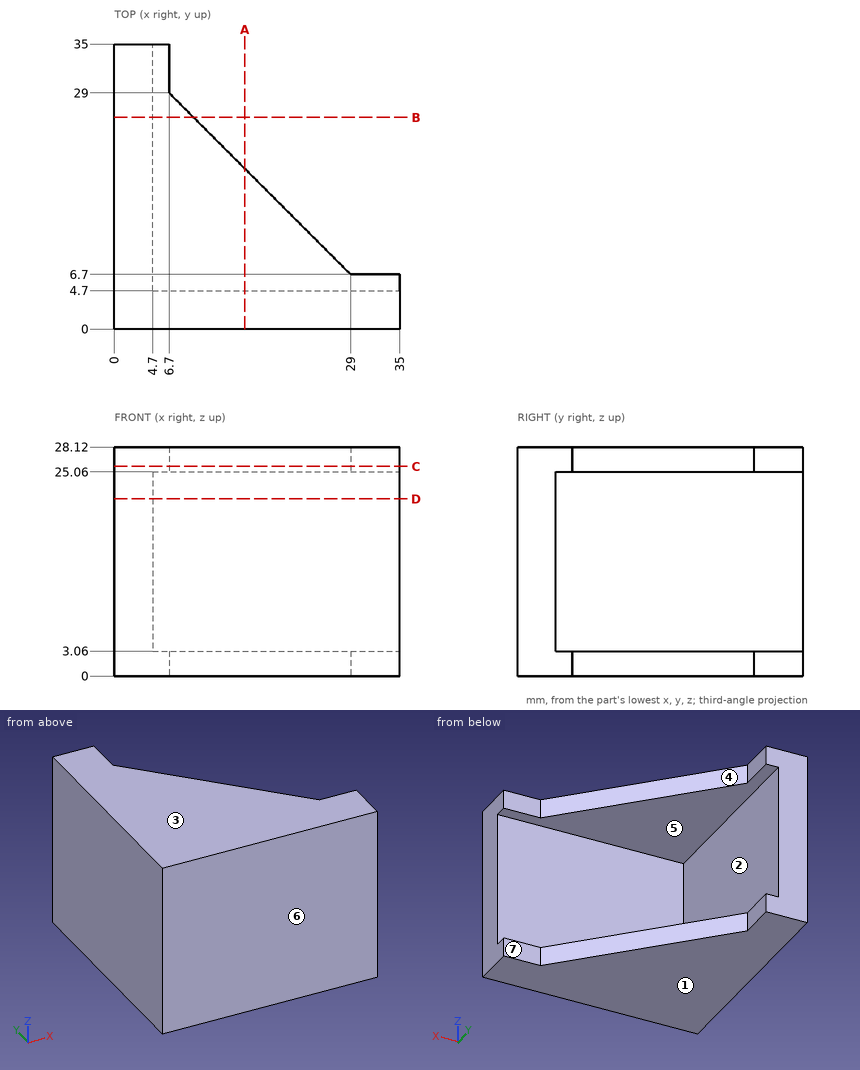
Could you check a few things on this drawing? It's one solid part, dimensions in mm from its lowest x, y, z. A direction names the side the tool comes from. Round coordinates to 2 decimals unless told otherwise and drop trailing zeros. Order: outer loops, then holes, each group sorted by start corner. A loop starts at its lowest first (then second) coordinate and runs counter-clockwise, first axis right, second up. Notation, with made-up numbers: M -25,19.25 L -14,19.25 A12 cw -14,23.25 Z; hole C 78,0.5 d8. An arc over 180 degrees is marked long. Return JSON: item names as keys, results as strings. Group by question number.
1. If we mould it in two halves opening along Z, with no side actions, what happens to the marked faces 1, 2, 3 and 4? For each: pulls with the +Z half, pulls with the -Z half, needs draft (parallel to the pull), parting line crosses it, or undercut.
2. If we section it at A-A on x = 16: List the corners of the cut face in (y, z) for me.
3. If we section it at B-B on y = 26: List the corners of the cut face in (x, z) for me, then the cut area to 3 significant figures.
4. I'm going to push flat-ended pins straight in: pin 1 Ø0.9 at (x, z) = (32, 1) entering from +Y; pin 2 Ø4 at (x, z) = (13.5, 4.5) entering from +Y; pin 3 Ø11 at (x, z) = (15.5, 17.5) entering from +Y. Where does each tip first touch, or does it pass through?
5. If we section it at D-D on z = 21.75: List the corners of the cut face in (x, y) for me, then the cut area to 3 significant figures.
6. On a 3-axis mill with a long thin cutter (end or side, diameter ignored), from which of +Z, -Z, +X, -X, +Y, -Y can I reach the whole of each face in a straight line? I mean the marked faces 5, 6 and 7. Say none if no direction works.
7. Please list where these lines run through material, in increasing order: probe 1 along Z at (x, y) = (15, 18.5); probe 2 along Y at (x, z) = (24, 23.25).
8. If we section it at C-C on z = 25.75: List the corners of the cut face in (x, y) for me, then the cut area to 3 significant figures.
Reply:
{
 "1": {"face 1": "pulls with the -Z half", "face 2": "undercut", "face 3": "pulls with the +Z half", "face 4": "needs draft"},
 "2": {"outline": "M 0,0 L 19.7,0 L 19.7,3.06 L 4.7,3.06 L 4.7,25.06 L 19.7,25.06 L 19.7,28.12 L 0,28.12 Z"},
 "3": {"outline": "M 0,0 L 9.7,0 L 9.7,3.06 L 4.7,3.06 L 4.7,25.06 L 9.7,25.06 L 9.7,28.12 L 0,28.12 Z", "area": "163 mm^2"},
 "4": {"pin 1": "y = 6.7", "pin 2": "y = 23.59", "pin 3": "y = 4.7"},
 "5": {"outline": "M 0,0 L 35,0 L 35,4.7 L 4.7,4.7 L 4.7,35 L 0,35 Z", "area": "307 mm^2"},
 "6": {"face 5": "+X, +Y", "face 6": "+Z, -Z, +X, -X, -Y", "face 7": "+Z, -Z, +X, +Y"},
 "7": {"probe 1": "0 to 3.06, 25.06 to 28.12", "probe 2": "0 to 4.7"},
 "8": {"outline": "M 0,0 L 35,0 L 35,6.7 L 29,6.7 L 6.7,29 L 6.7,35 L 0,35 Z", "area": "673 mm^2"}
}
